Model file for the job. Use its own axes, mm. Face numbers are marked on the shaded views. A direction names the side the tool comes from. Round coordinates to 2 decimals unless told otherwise and drop trailing zeros. Order: outer loops, then holes, each group sorted by start corner. A loop starts at its lowest first (then second) coordinate and runs counter-clockwise, first axis right, second up. Notation, with made-up numbers: (42, 68) - (90, 68) arc R18 ccw to (90, 96) - close; hole circle Ø7 at (-16.75, 31). An arc over 180 degrees is marked (long way). Write item = value, one per line. Start each with the question number.
from build123d import *

# Parameters (mm, degrees)
SKETCH1_W           = 70
SKETCH1_H           = 50
SKETCH1_R           = 3.1
BOSS_EXTRUDE1_DEPTH = 8
SKETCH3_W           = 70
SKETCH3_H           = 22
BOSS_EXTRUDE2_DEPTH = 4
BOSS_EXTRUDE3_DEPTH = 70


with BuildPart() as part:
    # Sketch1 → Boss-Extrude1 (new body)
    with BuildSketch(Plane.XY):
        with Locations((-11.480938416, -0.439882698)):
            Rectangle(SKETCH1_W, SKETCH1_H)
        with Locations((-26.480938416, 18.060117302)):
            Circle(SKETCH1_R, mode=Mode.SUBTRACT)
        with Locations((3.519061584, 18.060117302)):
            Circle(SKETCH1_R, mode=Mode.SUBTRACT)
        with Locations((-26.480938416, -18.939882698)):
            Circle(SKETCH1_R, mode=Mode.SUBTRACT)
        with Locations((3.519061584, -18.939882698)):
            Circle(SKETCH1_R, mode=Mode.SUBTRACT)
    extrude(amount=BOSS_EXTRUDE1_DEPTH)

    # Sketch3 → Boss-Extrude2 (add)
    with BuildSketch(Plane(origin=(0, 0, 0), x_dir=(-1, 0, 0), z_dir=(0, 0, -1))):
        with Locations((11.480938416, -0.439882698)):
            Rectangle(SKETCH3_W, SKETCH3_H)
    extrude(amount=BOSS_EXTRUDE2_DEPTH)

    # Sketch4 → Boss-Extrude3 (add)
    with BuildSketch(Plane.ZY.offset(46.480938416)):
        Polygon((-9, -0.439882698), (-4, -5.439882698), (-4, -0.439882698), (-4, 4.560117302), align=None)
    extrude(amount=-BOSS_EXTRUDE3_DEPTH)


solid = part.part
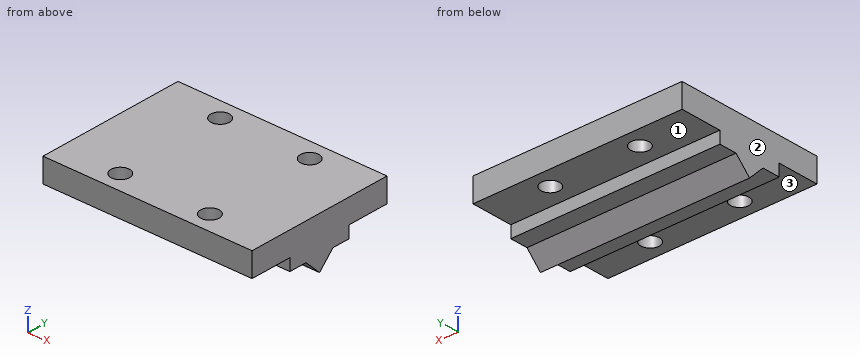
Item 1: Saw through at C-C, the plane x = -28. Give the cut face in (y, z).
Item 2: Drop flat-ended pins along their axis: pin 1 (12 mm diameter, centred on x = -7.5, y = -12.5, fed in from -Z); pin 2 (1 mm diameter, centred on x = 0, y = 15.5, fed in from -Z); pin 3 (3 mm diameter, centred on y = 6, z = -6, fed in from -X); pin 4 (10 mm diameter, centred on x = -21, z = -7, fed in from +Y). Give the stop position or say it passes through.
Item 3: Saw through at B-B, the plane z = 7.25. Give the cut face in (x, y), then the cut area to 3 significant figures.
Item 4: Saw through at D-D, the plane y = 9. Give the cut face in (x, z), then the cut area to 3 significant figures.
Item 5: Probe L1, parallel to X at y = -19, z = 4.75; L2, parallel to X at y = 16, z = 2.5; L3, parallel to Z at x = 11.5, y = -6. List the from-to ranges inside material, lowest first.
Item 6: Saw through at A-A, the plane x = -4. Give the cut face in (y, z), then the cut area to 3 significant figures.
Item 7: Which spindle directions (+Z, -Z, +X, -X, +Y, -Y) get a long thin tool onto all of the face, cutting with end or side? Do the marked faces 1, 2 and 3. Say none if no direction does.
Check sheet entries:
q1.outline = (-25.44, 0) - (-21.64, 0) - (-21.64, 8) - (-25.44, 8) - close; (-16.24, 0) - (-11.44, 0) - (-11.44, -4) - (-5.44, -4) - (-0.44, -9) - (4.56, -4) - (10.56, -4) - (10.56, 0) - (15.36, 0) - (15.36, 8) - (-16.24, 8) - close; (20.76, 0) - (24.56, 0) - (24.56, 8) - (20.76, 8) - close
q2.pin_1 = -4
q2.pin_2 = 0
q2.pin_3 = through
q2.pin_4 = 10.56
q3.outline = (-46.48, -25.44) - (23.52, -25.44) - (23.52, 24.56) - (-46.48, 24.56) - close; hole circle Ø6.2 at (-26.48, -18.94); hole circle Ø6.2 at (-26.48, 18.06); hole circle Ø6.2 at (3.52, -18.94); hole circle Ø6.2 at (3.52, 18.06)
q3.area = 3,380 mm2
q4.outline = (-46.48, -4) - (23.52, -4) - (23.52, 8) - (-46.48, 8) - close
q4.area = 840 mm2
q5.L1 = -46.48 to -29.58, -23.38 to 0.42, 6.62 to 23.52
q5.L2 = -46.48 to -28.8, -24.16 to 1.2, 5.84 to 23.52
q5.L3 = -4 to 8
q6.outline = (-25.44, 0) - (-11.44, 0) - (-11.44, -4) - (-5.44, -4) - (-0.44, -9) - (4.56, -4) - (10.56, -4) - (10.56, 0) - (24.56, 0) - (24.56, 8) - (-25.44, 8) - close
q6.area = 513 mm2
q7.face_1 = -Z, +X, -X, +Y
q7.face_2 = +Z, -Z, -X, +Y, -Y
q7.face_3 = -Z, +X, -X, -Y
